For this review, take the finished solid that the model builds, in its own axes (mm). A direction names the side the tool comes from. Round coordinates to 2 decimals unless told otherwise and drop trailing zeros. Write each loop counter-clockwise with the first axis right and the second up, starting at its lowest first coordinate (ties: lowest second). Pieces come first, ordered by that corner, then holes. Notation, with made-up numbers: (-12, 40.25) - (-7, 40.25) arc R35 cw to (-7, 73.25) - close; hole circle Ø9 at (58, -6.75). An arc over 180 degrees is marked (long way). One line per item, written item: value. Start each with the question number.
Q1. Mouldability with a two-part tool opening along Y and no side actions: class faces 1 (the face through (21, -17, 9)), 2 (the face through (-18.116, -17, 1)), 3 (the face through (2, 13.551, 1)) as +Y half, -Y half, draft (parallel to the pull), parting line (faces both ways), or undercut.
Q2. Clearance check with flat-ended pins moving along their axes: pin 1 Ø5 at (x, z) = (15.5, 17) entering from -Y; pin 2 Ø1.8 at (x, y) = (-11.12, 6.55) entering from +Z; pin 3 Ø9.5 at (x, z) = (14.5, 14) entering from +Y; pin 4 Ø2.5 at (y, z) = (-13, 25) entering from +X. State where each tip first meets the part, or that it passes through.
Q3. Add section B-B on y = -20. Write out the cut boundary in (x, z), and give its area (3 significant figures).
Q4. For probe 1 along Y at (x, z) = (13, 17); probe 2 along Z at (x, y) = (14.5, 2.5); probe 3 along Y at (x, z) = (5.5, 10), list the stretches that pass through material, from the lowest coordinate up.
Q5. Add section D-D on x = -4. Write out the cut boundary in (y, z), and give its area (3 significant figures).
Q6. Add section C-C on z = 11.25. Write out the cut boundary in (x, y).
Q7. Add section A-A on x = 2. Write out the cut boundary in (y, z), and give its area (3 significant figures).
Q8. Tool access review of faces 4 (the face through (10.01, -27.52, 5.6)), 5 (the face through (-0.515, -6.52, 15.874)), 6 (the face through (20.982, 4.923, 4.145)), 7 (the face through (17, -8.949, 18)), 8 (the face through (21.884, -17, 7)): name each direction out of +Z, -Z, +X, -X, +Y, -Y from which nothing blocks a thin tool from reaching the whole face with its end or side.
```python
from build123d import *

# Parameters (mm, degrees)
SKETCH1_W           = 40
SKETCH1_H           = 60
SKETCH1_R           = 1.5
BOSS_EXTRUDE1_DEPTH = 5
SKETCH3_W           = 23
SKETCH3_H           = 21
BOSS_EXTRUDE2_DEPTH = 22
CUT_EXTRUDE1_START  = -3
SKETCH4_W           = 2
SKETCH4_H           = 15
CUT_EXTRUDE1_DEPTH  = 15
FILLET1_R           = 3
FILLET2_R           = 2


with BuildPart() as part:
    # Sketch1 → Boss-Extrude1 (new body)
    with BuildSketch(Plane.XY):
        with Locations((1.884057971, -16.449275362)):
            Rectangle(SKETCH1_W, SKETCH1_H)
        with Locations((14.884057971, 6.550724638)):
            Circle(SKETCH1_R, mode=Mode.SUBTRACT)
        with Locations(Location((14.884057971, -39.449275362, 0), (0, 0, 180))):
            Circle(SKETCH1_R, mode=Mode.SUBTRACT)
        with Locations((-11.115942029, -39.449275362)):
            Circle(SKETCH1_R, mode=Mode.SUBTRACT)
        with Locations(Location((-11.115942029, 6.550724638, 0), (0, 0, 180))):
            Circle(SKETCH1_R, mode=Mode.SUBTRACT)
    extrude(amount=BOSS_EXTRUDE1_DEPTH)

    # Sketch3 → Boss-Extrude2 (add)
    with BuildSketch(Plane.XY.offset(5)):
        with Locations((10.384057971, -16.449275362)):
            Rectangle(SKETCH3_W, SKETCH3_H)
    extrude(amount=BOSS_EXTRUDE2_DEPTH)

    # Sketch4 → Cut-Extrude1 (cut)
    with BuildSketch(Plane.XZ.offset(26.949275362).offset(CUT_EXTRUDE1_START)):
        with Locations((20.884057971, 16.5)):
            Rectangle(SKETCH4_W, SKETCH4_H)
        Polygon((14.884057971, 24), (14.884057971, 14), (19.884057971, 9), (19.884057971, 24), align=None)
        Polygon((14.884057971, 27), (14.884057971, 24), (19.884057971, 24), (21.884057971, 24), (21.884057971, 27), align=None)
        Polygon((14.884057971, 24), (4.884057971, 24), (14.884057971, 14), align=None)
    extrude(amount=-CUT_EXTRUDE1_DEPTH, mode=Mode.SUBTRACT)

    # Fillet1
    fillet1_edges = [part.edges().sort_by_distance(p)[0] for p in [
        (21.884057971, -36.699275362, 5),
        (1.884057971, 13.550724638, 5),
        (21.884057971, 3.800724638, 5),
        (-18.115942029, -16.449275362, 5),
        (1.884057971, -46.449275362, 5),
    ]]
    fillet(fillet1_edges, radius=FILLET1_R)

    # Fillet2
    # the kernel refuses this fillet: 2 mm, written as the material it takes off along each edge
    with BuildSketch(Plane(origin=(0.884057971, -7.949275362, 25), x_dir=(-1, 0, 0), z_dir=(0, 0, 1))) as fillet2_piece_1_section:
        Polygon((0, 0), (FILLET2_R * 1.02, 0), (FILLET2_R * 1.02, -FILLET2_R * 1.02), (0, -FILLET2_R * 1.02), align=None)
    fillet2_piece_1 = extrude(amount=FILLET2_R * 1.02, mode=Mode.PRIVATE)
    fillet2_piece_1 = fillet2_piece_1 - Plane(origin=(0.884057971, -7.949275362, 25), x_dir=(0.7071067811865475, -0.7071067811865475, 0), z_dir=(0, 0, 1)) * Sphere(FILLET2_R, mode=Mode.PRIVATE)
    add(fillet2_piece_1, mode=Mode.SUBTRACT)
    with BuildSketch(Plane(origin=(0.884057971, -24.949275362, 25), x_dir=(-1, 0, 0), z_dir=(0, 0, 1))) as fillet2_piece_2_section:
        Polygon((0, 0), (FILLET2_R * 1.02, 0), (FILLET2_R * 1.02, FILLET2_R * 1.02), (0, FILLET2_R * 1.02), align=None)
    fillet2_piece_2 = extrude(amount=FILLET2_R * 1.02, mode=Mode.PRIVATE)
    fillet2_piece_2 = fillet2_piece_2 - Plane(origin=(0.884057971, -24.949275362, 25), x_dir=(0.7071067811865475, 0.7071067811865475, 0), z_dir=(0, 0, 1)) * Sphere(FILLET2_R, mode=Mode.PRIVATE)
    add(fillet2_piece_2, mode=Mode.SUBTRACT)
    with BuildSketch(Plane(origin=(-1.115942029, -5.949275362, 5), x_dir=(0, -1, 0), z_dir=(0, 0, 1))) as fillet2_piece_3:
        with BuildLine():
            CenterArc((FILLET2_R, FILLET2_R), FILLET2_R, 180, 90)
            Line((0, FILLET2_R), (0, 0))
            Line((0, 0), (FILLET2_R, 0))
        make_face()
    extrude(amount=20, mode=Mode.SUBTRACT)
    with BuildSketch(Plane(origin=(-1.115942029, -26.949275362, 5), x_dir=(0, 1, 0), z_dir=(0, 0, 1))) as fillet2_piece_4:
        with BuildLine():
            CenterArc((FILLET2_R, -FILLET2_R), FILLET2_R, 90, 90)
            Line((0, -FILLET2_R), (0, 0))
            Line((0, 0), (FILLET2_R, 0))
        make_face()
    extrude(amount=20, mode=Mode.SUBTRACT)
    with BuildSketch(Plane(origin=(0.884057971, -5.949275362, 27), x_dir=(0, -1, 0), z_dir=(1, 0, 0))) as fillet2_piece_5:
        with BuildLine():
            CenterArc((FILLET2_R, FILLET2_R), FILLET2_R, 180, 90)
            Line((0, FILLET2_R), (0, 0))
            Line((0, 0), (FILLET2_R, 0))
        make_face()
    extrude(amount=26, mode=Mode.SUBTRACT)
    with BuildSketch(Plane(origin=(-1.115942029, -24.949275362, 27), x_dir=(0, 0, -1), z_dir=(0, 1, 0))) as fillet2_piece_6:
        with BuildLine():
            CenterArc((FILLET2_R, -FILLET2_R), FILLET2_R, 90, 90)
            Line((0, -FILLET2_R), (0, 0))
            Line((0, 0), (FILLET2_R, 0))
        make_face()
    extrude(amount=17, mode=Mode.SUBTRACT)
    with BuildSketch(Plane(origin=(26.884057971, -26.949275362, 27), x_dir=(0, 0, -1), z_dir=(-1, 0, 0))) as fillet2_piece_7:
        with BuildLine():
            CenterArc((FILLET2_R, -FILLET2_R), FILLET2_R, 90, 90)
            Line((0, -FILLET2_R), (0, 0))
            Line((0, 0), (FILLET2_R, 0))
        make_face()
    extrude(amount=26, mode=Mode.SUBTRACT)
    # the kernel refuses this fillet: 2 mm, written as the material it adds along each edge
    with BuildSketch(Plane(origin=(-1.115942029, -24.949275362, 5), x_dir=(-1, 0, 0), z_dir=(0, 1, 0))) as fillet2_2_piece_1:
        with BuildLine():
            CenterArc((FILLET2_R, FILLET2_R), FILLET2_R, 180, 90)
            Line((0, FILLET2_R), (0, 0))
            Line((0, 0), (FILLET2_R, 0))
        make_face()
    extrude(amount=17)
    with BuildSketch(Plane(origin=(18.884057971, -26.949275362, 5), x_dir=(0, -1, 0), z_dir=(-1, 0, 0)), Plane(origin=(0.884057971, -5.949275362, 5), x_dir=(0, 1, 0), z_dir=(1, 0, 0))) as fillet2_2_piece_2:
        with BuildLine():
            CenterArc((FILLET2_R, FILLET2_R), FILLET2_R, 180, 90)
            Line((0, FILLET2_R), (0, 0))
            Line((0, 0), (FILLET2_R, 0))
        make_face()
    extrude(amount=18)
    with BuildSketch(Plane(origin=(18.884057971, -5.949275362, 2), x_dir=(-0.09638996566753259, 0, -0.9953436464450918), z_dir=(-0.9953436464450918, 0, 0.09638996566753259))) as fillet2_2_piece_3_section:
        with BuildLine():
            CenterArc((3 + FILLET2_R, -FILLET2_R), FILLET2_R, 90, 90)
            Line((3 + FILLET2_R, 0), (3, 0))
            Line((3, 0), (3, -FILLET2_R))
        make_face()
    fillet2_2_piece_3 = revolve(axis=Axis((18.884057971, -5.949275362, 2), (0, -1, 0)), revolution_arc=185.531326158, mode=Mode.PRIVATE)
    fillet2_2_piece_3 = split(fillet2_2_piece_3, bisect_by=Plane(origin=(21.104944702, -5.375674968, 0), z_dir=(0, 0, 1)), keep=Keep.TOP, mode=Mode.PRIVATE)
    fillet2_2_piece_3 = split(fillet2_2_piece_3, bisect_by=Plane(origin=(21.884057971, -5.375674968, 4.220886685), z_dir=(-1, 0, 0)), keep=Keep.TOP, mode=Mode.PRIVATE)
    add(fillet2_2_piece_3)
    with BuildSketch(Plane(origin=(18.884057971, -26.949275362, 2), x_dir=(-0.09638996566753259, 0, -0.9953436464450918), z_dir=(-0.9953436464450918, 0, 0.09638996566753259))) as fillet2_2_piece_4_section:
        with BuildLine():
            CenterArc((3 + FILLET2_R, FILLET2_R), FILLET2_R, 180, 90)
            Line((3 + FILLET2_R, 0), (3, 0))
            Line((3, 0), (3, FILLET2_R))
        make_face()
    fillet2_2_piece_4 = revolve(axis=Axis((18.884057971, -26.949275362, 2), (0, -1, 0)), revolution_arc=185.531326158, mode=Mode.PRIVATE)
    fillet2_2_piece_4 = split(fillet2_2_piece_4, bisect_by=Plane(origin=(21.104944699, -27.522875755, 0), z_dir=(0, 0, 1)), keep=Keep.TOP, mode=Mode.PRIVATE)
    fillet2_2_piece_4 = split(fillet2_2_piece_4, bisect_by=Plane(origin=(21.884057971, -27.522875755, 4.220886633), z_dir=(-1, 0, 0)), keep=Keep.TOP, mode=Mode.PRIVATE)
    add(fillet2_2_piece_4)
    with BuildSketch(Plane(origin=(0.884057971, -7.949275362, 5), x_dir=(-1, 0, 0), z_dir=(0, -1, 0))) as fillet2_2_piece_5:
        with BuildLine():
            CenterArc((2 + FILLET2_R, -FILLET2_R), FILLET2_R, 90, 90)
            Line((2, -FILLET2_R), (2, 0))
            Line((2, 0), (2 + FILLET2_R, 0))
        make_face()
    revolve(axis=Axis((0.884057971, -7.949275362, 5), (0, 0, -1)), revolution_arc=90)
    with BuildSketch(Plane(origin=(0.884057971, -24.949275362, 5), x_dir=(-1, 0, 0), z_dir=(0, 1, 0))) as fillet2_2_piece_6:
        with BuildLine():
            CenterArc((2 + FILLET2_R, FILLET2_R), FILLET2_R, 180, 90)
            Line((2, FILLET2_R), (2, 0))
            Line((2, 0), (2 + FILLET2_R, 0))
        make_face()
    revolve(axis=Axis((0.884057971, -24.949275362, 5), (0, 0, 1)), revolution_arc=90)


solid = part.part
```
Result set:
1. face 1: undercut
1. face 2: draft
1. face 3: +Y half
2. pin 1: stops at y = -26.95
2. pin 2: passes through
2. pin 3: stops at y = -5.95
2. pin 4: stops at x = 14.88
3. outline: (-18.12, 0) - (21.88, 0) - (21.88, 9) - (19.88, 9) - (4.88, 24) - (14.88, 24) - (14.88, 27) - (0.88, 27) arc R2 ccw to (-1.12, 25) - (-1.12, 7) arc R2 cw to (-3.12, 5) - (-15.12, 5) arc R3 ccw to (-18.12, 2) - close
3. area: 541 mm^2
4. probe 1: y = -26.95 to -23.95, -8.95 to -5.95
4. probe 2: z = 0 to 5
4. probe 3: y = -26.95 to -5.95
5. outline: (-46.45, 0) - (13.55, 0) - (13.55, 2) arc R3 ccw to (10.55, 5) - (-43.45, 5) arc R3 ccw to (-46.45, 2) - close
5. area: 296 mm^2
6. outline: (-1.12, -24.95) arc R2 ccw to (0.88, -26.95) - (21.88, -26.95) - (21.88, -23.95) - (17.63, -23.95) - (17.63, -8.95) - (21.88, -8.95) - (21.88, -5.95) - (0.88, -5.95) arc R2 ccw to (-1.12, -7.95) - close
7. outline: (-46.45, 0) - (13.55, 0) - (13.55, 2) arc R3 ccw to (10.55, 5) - (-3.95, 5) arc R2 cw to (-5.95, 7) - (-5.95, 25) arc R2 ccw to (-7.95, 27) - (-24.95, 27) arc R2 ccw to (-26.95, 25) - (-26.95, 7) arc R2 cw to (-28.95, 5) - (-43.45, 5) arc R3 ccw to (-46.45, 2) - close
7. area: 758 mm^2
8. face 4: +Z, +X, -X, -Y
8. face 5: +Z, -X, +Y
8. face 6: +Z, +X, +Y
8. face 7: +X
8. face 8: +Z, -Z, +X, +Y, -Y
